Read the model definition and answer for the solid it produces. Units are mm, in the model's axes. Face numbers are marked on the shaded views. A direction names the side the tool comes from. Coordinates: 2 decimals unless noted, no trailing zeros. Order: outer loops, then holes, each group sorted by start corner. A loop starts at its lowest first (then second) coordinate and runs counter-clockwise, first axis right, second up. Notation, with made-up numbers: (89, -6.5) - (117, -6.5) arc R15 ccw to (117, -2.5) - close; hole circle Ø4 at (-2.5, -18.75). An arc over 180 degrees is marked (long way). Answer as a JSON object with one key per item and string values. Group by question number.
from build123d import *

# Parameters (mm, degrees)
F2_DEPTH       = 7.5
F3_R           = 13
F4_DEPTH       = 15.001
F5_R           = 7.49999
F7_D           = 5
F7_CBORE_D     = 10
F7_CBORE_DEPTH = 1
F9_DEPTH       = 2


# Not quite as in the source:
# - a fillet or chamfer is up to 0.001 mm smaller than in the source, because OpenCascade refuses the exact size


with BuildPart() as f2:
    # F1 (on Front) → F2 (new body, symmetric)
    with BuildSketch(Plane.XZ):
        with BuildLine():
            Line((-37.5, 0), (0, 0))
            Line((0, 0), (37.5, 0))
            Line((37.5, 0), (37.5, 4))
            Line((37.5, 4), (10.9544511501, 4))
            ThreePointArc((10.9544511501, 4), (9.0757782768, 5.3140056594), (9.6656921913, 7.5294117647))
            ThreePointArc((9.6656921913, 7.5294117647), (14.0900465494, 24.1449575543), (0, 34))
            ThreePointArc((0, 34), (-14.0900465494, 24.1449575543), (-9.6656921913, 7.5294117647))
            ThreePointArc((-9.6656921913, 7.5294117647), (-9.0757782768, 5.3140056594), (-10.9544511501, 4))
            Line((-10.9544511501, 4), (-37.5, 4))
            Line((-37.5, 4), (-37.5, 0))
        make_face()
    extrude(amount=F2_DEPTH, both=True)

    # F3 (on face) → F4 (cut, through all)
    with BuildSketch(Plane.XZ.offset(7.5)):
        with Locations((0, 19)):
            Circle(F3_R)
    extrude(amount=-F4_DEPTH, mode=Mode.SUBTRACT)

    # F5 (radius 7.5 in the source; OpenCascade refuses exactly that, so slightly less here)
    f5_edges = [f2.edges().sort_by_distance(p)[0] for p in [
        (37.5, -7.5, 2),
        (37.5, 7.5, 2),
        (-37.5, -7.5, 2),
        (-37.5, 7.5, 2),
    ]]
    fillet(f5_edges, radius=F5_R)

    # F7 (through all)
    with Locations(Plane.XY.offset(4)):
        with Locations((30, 0), (-30, 0)):
            CounterBoreHole(F7_D / 2, F7_CBORE_D / 2, F7_CBORE_DEPTH)

    # F8 (on Front) → F9 (join, symmetric)
    with BuildSketch(Plane.XZ):
        with BuildLine():
            Line((10.9544511501, 4), (24, 4))
            Line((24, 4), (13.4831460674, 25.5730337079))
            ThreePointArc((13.4831460674, 25.5730337079), (14.6751576274, 15.8952055444), (9.6656921913, 7.5294117647))
            ThreePointArc((9.6656921913, 7.5294117647), (9.0757782768, 5.3140056594), (10.9544511501, 4))
        make_face()
    extrude(amount=F9_DEPTH, both=True)

    # F10: F2 across plane


with BuildPart() as f2_1:
    add(f2.part)
    add(f2.part.mirror(Plane.YZ))


solid = f2_1.part
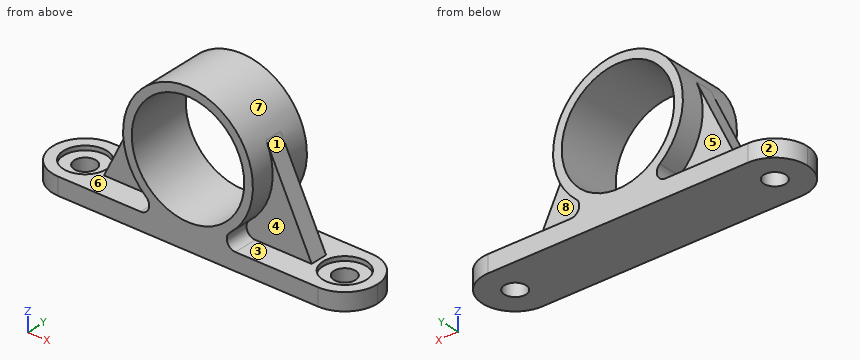
1. For the marked faces 4, 5, 6, 7 and 8, determine the directions among +Z, -Z, +X, -X, +Y, -Y from which every point of the face is accessible in a straight line to the end or side of a thin tool.
2. Straight lines are drawn through the part: L1, parallel to X at y = 0, z = 3.3; L2, parallel to Y at x = -30, z = 1; L3, parallel to Z at x = 0, y = -2. For each, find the intervals that lie inside material, in ascending order.
3. A cutting plane is placed at A-A on x = 0. Write down the section's boundary in (y, z), and give its area (3 significant figures).
4. A cutting plane is placed at D-D on z = 21.5. Write down the section's boundary in (x, y), and give its area (3 significant figures).
5. Given pin 1 (8 mm diameter, centred on x = -29, y = -0.5, fed in from +Z); pin 2 (4.5 mm diameter, centred on x = -17.5, z = 12, fed in from +Y); pin 3 (6 mm diameter, centred on x = 30, y = 0, fed in from +Z), each flat-ended and moving along its own axis, determine where each tip first touches the part or whether it passes through.
6. For a pull along Z with two mould halves and no side action, classify the marked faces 1, 2 and 3 as pulls with the +Z half, pulls with the -Z half, needs draft (parallel to the pull), parting line crosses it, or undercut.
7. A cutting plane is placed at C-C on x = -8. Write down the section's boundary in (y, z).
8. A cutting plane is placed at B-B on z = 14. Write down the section's boundary in (x, y) (3 decimals).
Derived:
{
 "1": {"face 4": "+X, -Y", "face 5": "-X, +Y", "face 6": "-X", "face 7": "none", "face 8": "+X, +Y"},
 "2": {"L1": "x = -37.5 to -35, -25 to 25, 35 to 37.5", "L2": "y = -7.5 to -2.5, 2.5 to 7.5", "L3": "z = 0 to 6, 32 to 34"},
 "3": {"outline": "(-7.5, 0) - (7.5, 0) - (7.5, 6) - (-7.5, 6) - close; (-7.5, 32) - (7.5, 32) - (7.5, 34) - (-7.5, 34) - close", "area": "120 mm2"},
 "4": {"outline": "(-15.47, -2) - (-14.79, -2) - (-14.79, -7.5) - (-12.76, -7.5) - (-12.76, 7.5) - (-14.79, 7.5) - (-14.79, 2) - (-15.47, 2) - close; (12.76, -7.5) - (14.79, -7.5) - (14.79, -2) - (15.47, -2) - (15.47, 2) - (14.79, 2) - (14.79, 7.5) - (12.76, 7.5) - close", "area": "66.4 mm2"},
 "5": {"pin 1": "stops at z = 4", "pin 2": "stops at y = 2", "pin 3": "stops at z = 3"},
 "6": {"face 1": "pulls with the +Z half", "face 2": "needs draft", "face 3": "undercut"},
 "7": {"outline": "(-7.5, 0) - (7.5, 0) - (7.5, 8.75) - (-7.5, 8.75) - close; (-7.5, 29.25) - (7.5, 29.25) - (7.5, 31.69) - (-7.5, 31.69) - close"},
 "8": {"outline": "(-19.125, -2) - (-14.142, -2) - (-14.142, -7.5) - (-12, -7.5) - (-12, 7.5) - (-14.142, 7.5) - (-14.142, 2) - (-19.125, 2) - close; (12, -7.5) - (14.142, -7.5) - (14.142, -2) - (19.125, -2) - (19.125, 2) - (14.142, 2) - (14.142, 7.5) - (12, 7.5) - close"}
}
